Could you check a few things on this model? Use its own coordinates, in mm. Face numbers are marked on the shaded views. A direction names the side the tool comes from. Give positions to 0.01 mm unless a question says otherwise; leave off trailing zeros. Order: outer loops, then holes, each group sorted by start corner. A loop starts at its lowest first (then second) coordinate and runs counter-clockwise, first axis right, second up. Notation, with made-up numbers: (20.5, 51) -> (59.5, 51) arc R22 ccw to (59.5, 61) -> close; hole circle Ø3 at (12, 38.5). An arc over 180 degrees is marked (long way). Answer as CSV lines item,"result". Start each with the question number.
(1) Will these pins go through, and if not, where does the flat tip stop? pin 1 Ø2.5 at (x, z) = (20.66, -5) entering from +Y; pin 2 Ø2 at (x, z) = (36, -6.5) entering from -Y; pin 3 Ø4 at (x, z) = (54.5, 2.5) entering from -Y; pin 4 Ø3.5 at (x, z) = (59.34, -5) entering from -Y.
(2) We'd pull the mould along X, two halves only. Please class the marked faces 3, 4, 5 and 6: released by +X, released by -X, zero draft, split by the parting line, or undercut.
(3) On a 3-axis mill with a long thin cutter (end or side, diameter ignored), from which of +Z, -Z, +X, -X, +Y, -Y can I reach the whole of each face in a straight line? I mean the marked faces 1 and 2. Say none if no direction works.
(4) I want a section at A-A (x = 78). Please give me the cut outline in (y, z).
(5) I want a section at B-B (y = 8). Give the number of separate pieces and of enclosed holes in the cut face, plus the area to 3 significant figures.
(6) I want a section at C-C (z = 2.25). Please give me the cut outline in (x, y), plus the area to 3 significant figures.
(7) I need wall thicknesses on L1, parallel to X at y = 13.85, z = -5; L2, parallel to Z at x = 9, y = 1.75; L3, parallel to Z at x = 59.34, y = 11.95. Which ranges of each line are inside material? Lowest first, please.
(8) I want a section at D-D (y = 3.5). Please give me the cut outline in (x, z), plus the area to 3 significant figures.
Autodesk Inventor part; units mm, degrees
ref_plane "YZ Plane" through (0, 0, 0) normal (1, 0, 0) x (0, 1, 0)
ref_plane "XZ Plane" through (0, 0, 0) normal (0, 1, 0) x (-1, 0, 0)
ref_plane "XY Plane" through (0, 0, 0) normal (0, 0, 1) x (1, 0, 0)
sketch "Boceto1" plane through (0, 0, 0) normal (0, 1, 0) x (-1, 0, 0)
  line L0 (0, 0) -> (-80, 0)
  line L1 (-80, 0) -> (-80, -10)
  line L2 (-80, -10) -> (0, -10)
  line L3 (0, -10) -> (0, 0)
  line L4 (5, 0) -> (5, 5)
  line L5 (-80, -10) -> (-80, -15)
  line L6 (-80, -15) -> (-85, -15)
  line L7 (5, 5) -> (-85, 5)
  line L8 (-85, 5) -> (-85, -15)
  line L9 (-85, -15) -> (5, -15)
  line L10 (5, -15) -> (5, 5)
  dimension "d1" = 10
  dimension "d2" = 5
  dimension "d3" = 5
  dimension "d5" = 5
extrude "Extrusión1" add sketch "Boceto1" along normal blind 15
sketch "Boceto2" plane through (0, 15, 0) normal (0, 1, 0) x (1, 0, 0)
  line L0 (80, 10) -> (80, 0)
  line L1 (80, 0) -> (0, 0)
  line L2 (0, 0) -> (0, 10)
  line L3 (0, 10) -> (80, 10)
  line L4 (80, 10) -> (80, 0)
extrude "Extrusión2" add sketch "Boceto2" against normal blind 5
sketch "Boceto3" plane through (-5, 0, 5) normal (0, 0, 1) x (1, 0, 0)
  line L0 (90, 15) -> (90, 9)
  line L1 (90, 0) -> (90, 15)
  line L2 (90, 9) -> (50, 9)
  line L3 (50, 9) -> (50, -31)
  circle A0 centre (50, -31) radius 40
  point P0 (5, 0)
  dimension "d10" = 6
  dimension "d11" = 40
  dimension "d12" = 40
extrude "Extrusión3" cut sketch "Boceto3" against normal blind 21
sketch "Boceto4" plane through (0, 10, 0) normal (0, -1, 0) x (1, 0, 0)
  line L0 (0, 0) -> (0, -5)
  line L1 (0, 0) -> (0, -10)
  line L2 (0, -5) -> (80, -5)
  line L3 (80, -10) -> (80, 0)
  line L4 (80, -5) -> (59.34, -5)
  line L5 (0, -5) -> (20.66, -5)
  dimension "d15" = 5
  dimension "d16" = 20.66
  dimension "d17" = 20.66
hole "Agujero1" at (20.66, 10, -5) at (59.34, 10, -5) direction (0, 1, 0) diameter 3 end through all countersink diameter 5 countersink angle 90
sketch "Boceto5" plane through (85, 15, -15) normal (0, 0, -1) x (-1, 0, 0)
  line L0 (90, -15) -> (90, 0)
  line L1 (90, 0) -> (83, 0)
  line L2 (0, 0) -> (90, 0)
  line L3 (83, 0) -> (83, -7)
  point P0 (85, -15)
  dimension "d25" = 7
  dimension "d26" = 7
sketch "Boceto6" plane through (85, 15, -15) normal (0, 0, -1) x (-1, 0, 0)
  line L0 (0, 0) -> (90, 0)
  line L1 (0, 0) -> (0, -7)
  line L2 (0, -15) -> (0, 0)
  line L3 (0, -7) -> (7, -7)
  circle A0 centre (7, -7) radius 1.6
  line L4 (90, 0) -> (83, 0)
  line L5 (83, 0) -> (83, -7)
  circle A1 centre (83, -7) radius 1.6
  point P0 (85, -15)
  dimension "d27" = 7
  dimension "d28" = 7
  dimension "d29" = 3.2
  dimension "d30" = 7
  dimension "d31" = 7
  dimension "d32" = 3.2
extrude "Extrusión4" cut sketch "Boceto6" against normal blind 28.75
properties part number "Base Ventilador"
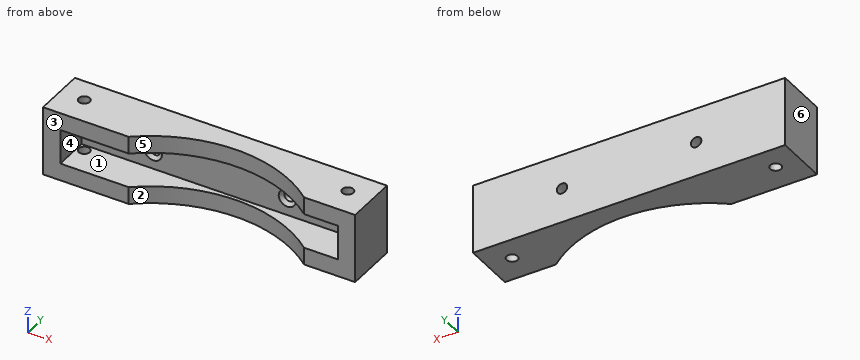
Final values:
1,pin 1,"through"
1,pin 2,"y = 10"
1,pin 3,"y = 7.31"
1,pin 4,"y = 10.75"
2,face 3,"zero draft"
2,face 4,"undercut"
2,face 5,"undercut"
2,face 6,"released by -X"
3,face 1,"-Y"
3,face 2,"+Z, -Z, -Y"
4,outline,"(0, -15) -> (6.4, -15) -> (6.4, -10) -> (0, -10) -> close; (0, 0) -> (6.4, 0) -> (6.4, 5) -> (0, 5) -> close; (9.6, -15) -> (15, -15) -> (15, 5) -> (9.6, 5) -> (9.6, 0) -> (10, 0) -> (10, -10) -> (9.6, -10) -> close"
5,separate pieces,"6"
5,enclosed holes,"0"
5,area,"758 mm²"
6,outline,"(-5, 0) -> (19.72, 0) arc R40 cw to (70.28, 0) -> (85, 0) -> (85, 15) -> (-5, 15) -> close; hole circle Ø3.2 at (2, 8); hole circle Ø3.2 at (78, 8)"
6,area,"1,020 mm²"
7,L1,"-5 to 19.16, 22.16 to 57.84, 60.84 to 85"
7,L2,"-15 to -10, 0 to 5"
7,L3,"-15 to -6.5, -3.5 to 5"
8,outline,"(-5, -15) -> (24.76, -15) -> (24.76, -10) -> (0, -10) -> (0, 0) -> (24.76, 0) -> (24.76, 5) -> (-5, 5) -> close; (65.24, -15) -> (85, -15) -> (85, 5) -> (65.24, 5) -> (65.24, 0) -> (80, 0) -> (80, -10) -> (65.24, -10) -> close"
8,area,"595 mm²"
